Check sheet for the modelled part. Datum: model origin and axes. Units: mm. A direction names the side the tool comes from. Coordinates: 2 decimals unless noted, no trailing zeros. Loops run counter-clockwise (first coordinate to the right, second up) from the corner with the lowest first, then second, coordinate; pieces in that order, holes last.
```python
from build123d import *

# Parameters (mm, degrees)
SKETCH1_W                      = 12.7
SKETCH1_H                      = 19.05
SKETCH1_W_2                    = 25.4
BOSS_EXTRUDE1_DEPTH            = 6.35
SKETCH1_3_W                    = 25.4
SKETCH1_3_H                    = 19.05
BOSS_EXTRUDE2_DEPTH            = 38.1
F_8_CLEARANCE_HOLE1_AT_2_COUNT = 2
F_8_CLEARANCE_HOLE1_AT_2_PITCH = 38.1
CHAMFER1_SIZE                  = 1.27
CHAMFER2_SIZE                  = 0.254


with BuildPart() as part:
    # Sketch1 → Boss-Extrude1 (new body)
    with BuildSketch(Plane(origin=(0, 0, 0), x_dir=(1, 0, 0), z_dir=(0, 1, 0))):
        with Locations((-19.05, 0)):
            Rectangle(SKETCH1_W, SKETCH1_H)
        Rectangle(SKETCH1_W_2, SKETCH1_H)
        with Locations((19.05, 0)):
            Rectangle(SKETCH1_W, SKETCH1_H)
    extrude(amount=BOSS_EXTRUDE1_DEPTH)

    # Sketch1_3 → Boss-Extrude2 (add)
    with BuildSketch(Plane(origin=(0, 0, 0), x_dir=(1, 0, 0), z_dir=(0, 1, 0))):
        Rectangle(SKETCH1_3_W, SKETCH1_3_H)
    extrude(amount=BOSS_EXTRUDE2_DEPTH)

    # Sketch4 → 3_8-16 Tapped Hole1 (revolve, cut)
    with BuildSketch(Plane(origin=(0, 25.4, 9.525), x_dir=(0, -1, 0), z_dir=(1, 0, 0))):
        Polygon((0, 0), (0, 19.05), (4.826, 19.05), (3.96875, 18.19275), (3.96875, 0.85725), (4.826, 0), align=None)
    revolve(axis=Axis((0, 25.4, 15.875), (0, 0, -1)), mode=Mode.SUBTRACT)

    # Sketch8 → 8 Clearance Hole1 (revolve, cut)
    with BuildSketch(Plane(origin=(-19.05, 6.35, 0), x_dir=(0, 0, 1), z_dir=(1, 0, 0))):
        Polygon((0, 0), (0, 6.35), (2.8829, 6.35), (2.2479, 5.715), (2.2479, 0.635), (2.8829, 0), align=None)
    f_8_clearance_hole1 = revolve(axis=Axis((-19.05, 12.7, 0), (0, -1, 0)), mode=Mode.SUBTRACT)

    # 8 Clearance Hole1 at 2: 8 Clearance Hole1 ×2
    with Locations(*[(i * F_8_CLEARANCE_HOLE1_AT_2_PITCH, 0, 0) for i in range(1, F_8_CLEARANCE_HOLE1_AT_2_COUNT)]):
        add(f_8_clearance_hole1, mode=Mode.SUBTRACT)

    # Chamfer1
    chamfer1_edges = [part.edges().sort_by_distance(p)[0] for p in [
        (25.4, 6.35, 0),
        (-19.05, 6.35, -9.525),
        (19.05, 6.35, 9.525),
        (19.05, 6.35, -9.525),
        (-25.4, 6.35, 0),
        (0, 38.1, -9.525),
        (-12.7, 38.1, 0),
        (0, 38.1, 9.525),
        (12.7, 38.1, 0),
        (-19.05, 6.35, 9.525),
    ]]
    chamfer(chamfer1_edges, length=CHAMFER1_SIZE)

    # Chamfer2
    chamfer2_edges = [part.edges().sort_by_distance(p)[0] for p in [
        (-25.4, 0, 0),
        (0, 0, -9.525),
        (-12.7, 21.59, -9.525),
        (-12.7, 21.59, 9.525),
        (25.4, 0, 0),
        (12.7, 21.59, -9.525),
        (25.4, 2.54, -9.525),
        (-25.4, 2.54, -9.525),
        (0, 0, 9.525),
        (12.7, 21.59, 9.525),
        (25.4, 2.54, 9.525),
        (-25.4, 2.54, 9.525),
    ]]
    chamfer(chamfer2_edges, length=CHAMFER2_SIZE)


solid = part.part
```
1) Depth check by flat-ended pin: pin 1 (5.5 mm diameter, centred on y = 13.5, z = 0.5, fed in from +X); pin 2 (12 mm diameter, centred on x = 20, y = 26, fed in from -Z); pin 3 (9.5 mm diameter, centred on y = 22.5, z = 1, fed in from -X); pin 4 (1 mm diameter, centred on x = 4, z = 0, fed in from -Y). Enter the tip coordinate at first touch or a pass-through.
Answer sheet:
pin 1: stops at x = 12.7
pin 2: passes through
pin 3: stops at x = -12.7
pin 4: stops at y = 0
2) Set-up check for faces 1 (the flat face through (18.77, 5.724, 8.881)), 2 (the flat face through (16, 6.35, 0)), 3 (the flat face through (0, 0, 0)), 4 (the flat face through (-18.949, 5.724, 8.881)), 5 (the flat face through (0, 18, -9.525)): record each of +Z, -Z, +X, -X, +Y, -Y from which the full face is reachable in a straight line by a thin tool's end or side.
Answer sheet:
face 1: +Z, +X, +Y
face 2: +Z, -Z, +X, +Y
face 3: +Z, -Z, +X, -X, -Y
face 4: +Z, -X, +Y
face 5: -Z, +X, -X, +Y, -Y
3) Section check D-D on y = 3. Enter the section's corners in (x, z) (3 decimals), plus the area to 3 significant figures.
Answer sheet:
outline: (-25.4, -9.271) - (-25.146, -9.525) - (25.146, -9.525) - (25.4, -9.271) - (25.4, 9.271) - (25.146, 9.525) - (-25.146, 9.525) - (-25.4, 9.271) - close; hole circle Ø4.496 at (-19.05, 0); hole circle Ø4.496 at (19.05, 0)
area: 936 mm2
4) Section check B-B on y = 25.4. Enter the section's corners in (x, z) (3 decimals), plus the area to 3 significant figures.
Answer sheet:
outline: (-12.7, -9.271) - (-12.446, -9.525) - (-4.826, -9.525) - (-3.969, -8.668) - (-3.969, 8.668) - (-4.826, 9.525) - (-12.446, 9.525) - (-12.7, 9.271) - close; (3.969, -8.668) - (4.826, -9.525) - (12.446, -9.525) - (12.7, -9.271) - (12.7, 9.271) - (12.446, 9.525) - (4.826, 9.525) - (3.969, 8.668) - close
area: 331 mm2
5) Mould release check, pull along Z, two halves, no side actions. Record for faces 6 (the cylindrical face through (-21.28, 3.21, -0.29)), 7 (the flat face through (0, 38.1, 0)), 8 (the flat face through (18.949, 5.706, -8.899)): +Z half, -Z half, draft (parallel to the pull), parting line (faces both ways), or undercut.
Answer sheet:
face 6: undercut
face 7: draft
face 8: -Z half
6) Scan lines: line 1 (X direction, y = 3.85, z = 0); line 2 (Z direction, x = 19.05, y = 1.8) (3 decimals); line 3 (X direction, y = 25.4, z = 3.25). Record each from-to range of solid material in increasing order.
Answer sheet:
line 1: x = -25.4 to -21.3, -16.8 to 16.8, 21.3 to 25.4
line 2: z = -9.525 to -2.248, 2.248 to 9.525
line 3: x = -12.7 to -3.97, 3.97 to 12.7
7) Section check C-C on x = -19.05. Enter the section's corners in (y, z) (3 decimals).
Answer sheet:
outline: (0, -9.271) - (0.254, -9.525) - (5.08, -9.525) - (6.35, -8.255) - (6.35, -2.883) - (5.715, -2.248) - (0.635, -2.248) - (0, -2.883) - close; (0, 2.883) - (0.635, 2.248) - (5.715, 2.248) - (6.35, 2.883) - (6.35, 8.255) - (5.08, 9.525) - (0.254, 9.525) - (0, 9.271) - close
8) Section check A-A on z = 0. Give the number of separate pieces and of enclosed holes in the cut face, plus the area to 3 significant figures.
Answer sheet:
separate pieces: 3
enclosed holes: 1
area: 1,020 mm2
